Check sheet for the drawn part. Datum: minimum x, y, z corner. Units: mm. A direction names the side the tool comes from. Give positions to 0.01 mm unless a question says otherwise; leave off trailing zeros. Loops run counter-clockwise (first coordinate to the right, second up) from the corner with the lowest first, then second, coordinate; pieces in that order, holes last.
1. Cross-section at B-B, the plane y = 50. Record the cut outline in (x, z), plus the area to 3 significant figures.
2. Release check for a two-part mould opening along Y. For the marked faces 1, 2 and 3 record: +Y half, -Y half, draft (parallel to the pull), parting line (faces both ways), or undercut.
3. Cross-section at A-A, the plane z = 17.5. Record the cut outline in (x, y), plus the area to 3 significant figures.
4. Tool access check on the marked faces 4 and 5. Record the directions out of +Z, -Z, +X, -X, +Y, -Y that give a thin tool (end or side, any length) a straight path to the whole face; none if there is none.
5. Material ranges on L1, parallel to Y at x = 100, z = 16.5; L2, parallel to X at y = 77, z = 21.75 (1 decimal); L3, parallel to X at y = 34, z = 7, recorded low to high.
6. Go/stop test with flat-tipped pins: pin 1 Ø5 at (x, y) = (24.5, 46) entering from +Z; pin 2 Ø1 at (x, y) = (23, 79.5) entering from -Z. Record where each tip stops, or that it passes through.
7. Cross-section at D-D, the plane z = 5.25. Record the cut outline in (x, y), plus the area to 3 significant figures.
8. Cross-section at C-C, the plane x = 100. Record the cut outline in (y, z).
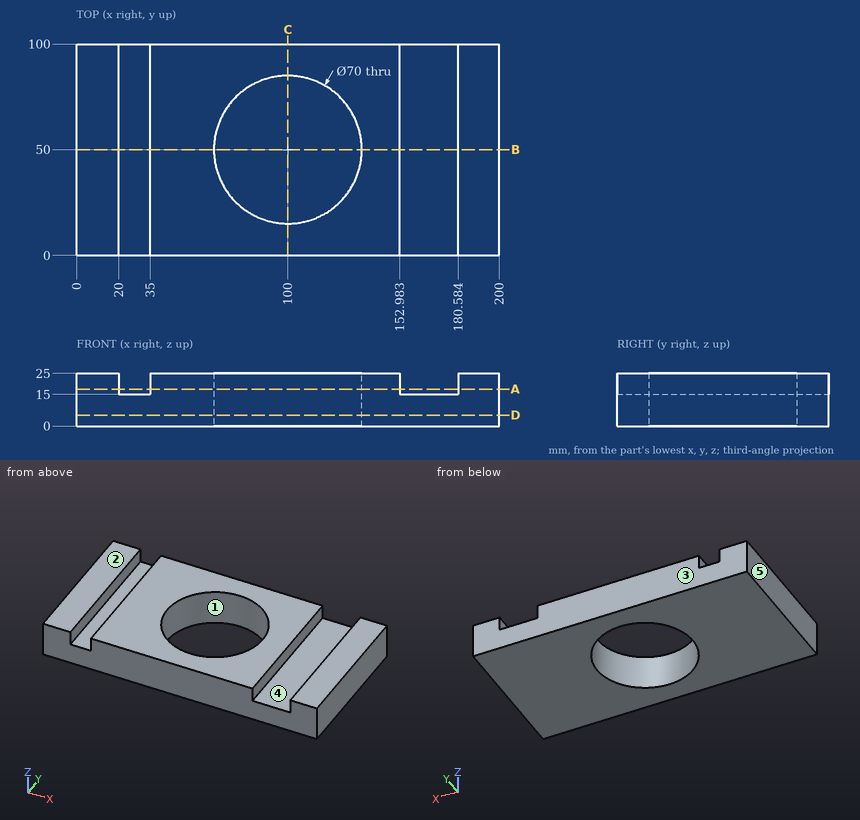
Result:
1. outline: (0, 0) - (65, 0) - (65, 25) - (35, 25) - (35, 15) - (20, 15) - (20, 25) - (0, 25) - close; (135, 0) - (200, 0) - (200, 25) - (180.58, 25) - (180.58, 15) - (152.98, 15) - (152.98, 25) - (135, 25) - close
1. area: 2,820 mm2
2. face 1: undercut
2. face 2: draft
2. face 3: +Y half
3. outline: (0, 0) - (20, 0) - (20, 100) - (0, 100) - close; (35, 0) - (152.98, 0) - (152.98, 100) - (35, 100) - close; (180.58, 0) - (200, 0) - (200, 100) - (180.58, 100) - close; hole circle Ø70 at (100, 50)
3. area: 11,900 mm2
4. face 4: +Z, +Y, -Y
4. face 5: +Z, -Z, -X, +Y, -Y
5. L1: y = 0 to 15, 85 to 100
5. L2: x = 0 to 20, 35 to 77.7, 122.3 to 153, 180.6 to 200
5. L3: x = 0 to 68.87, 131.13 to 200
6. pin 1: stops at z = 15
6. pin 2: stops at z = 0
7. outline: (0, 0) - (200, 0) - (200, 100) - (0, 100) - close; hole circle Ø70 at (100, 50)
7. area: 16,200 mm2
8. outline: (0, 0) - (15, 0) - (15, 25) - (0, 25) - close; (85, 0) - (100, 0) - (100, 25) - (85, 25) - close
